CAD build for the part. Positions are in the model's coordinates, mm. Face numbers are marked on the shaded views. Give positions to 0.01 mm unless a question says otherwise; leave off trailing zeros. Loops run counter-clockwise (first coordinate to the right, second up) from the corner with the lowest first, then second, coordinate; pieces in that order, holes last. Notation, with made-up numbers: M -35,86 L 16,86 A12 ccw 16,106 Z; hole C 74.25,-38.75 d7. An arc over 180 degrees is marked long. One line per question, with ' | ' between items.
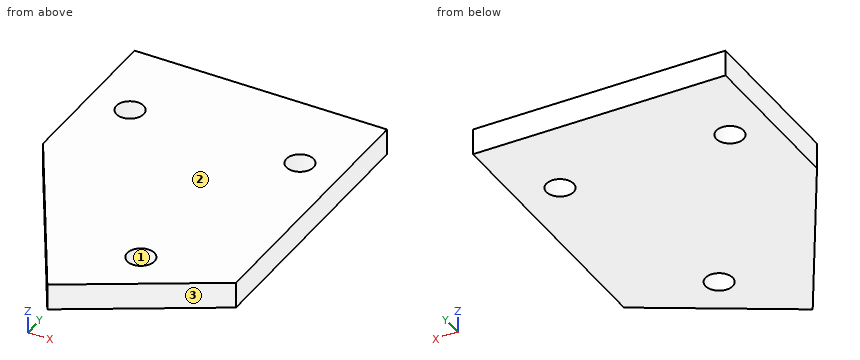
```python
from build123d import *

# Parameters (mm, degrees)
SKETCH1_R           = 1.65
BOSS_EXTRUDE1_DEPTH = 3.175


with BuildPart() as part:
    # Sketch1 → Boss-Extrude1 (new body)
    with BuildSketch(Plane.XY):
        Polygon((0, 0), (13.273502692, -22.990381057), (30.594010768, -12.990381057), (30.594010768, 20), (0, 20), align=None)
        with Locations((19.43375673, -13.660254038)):
            Circle(SKETCH1_R, mode=Mode.SUBTRACT)
        with Locations((5, 10)):
            Circle(SKETCH1_R, mode=Mode.SUBTRACT)
        with Locations((25.594010768, 10)):
            Circle(SKETCH1_R, mode=Mode.SUBTRACT)
    extrude(amount=BOSS_EXTRUDE1_DEPTH)


solid = part.part
```
Item 1: Saw through at A-A on y = 10. Give the cut face in (x, z) (3 decimals).
Conclusion:
outline: M 0,0 L 3.35,0 L 3.35,3.175 L 0,3.175 Z; M 6.65,0 L 23.944,0 L 23.944,3.175 L 6.65,3.175 Z; M 27.244,0 L 30.594,0 L 30.594,3.175 L 27.244,3.175 Z
Item 2: Saw through at D-D on y = -19. Give the cut face in (x, z) (3 decimals).
Conclusion:
outline: M 10.97,0 L 20.185,0 L 20.185,3.175 L 10.97,3.175 Z
Item 3: Saw through at B-B on z = 1.8. Give the cut face in (x, y), and give its area (3 significant figures).
Conclusion:
outline: M 0,0 L 13.27,-22.99 L 30.59,-12.99 L 30.59,20 L 0,20 Z; hole C 5,10 d3.3; hole C 19.43,-13.66 d3.3; hole C 25.59,10 d3.3 | area: 1,050 mm²
Item 4: Saw through at C-C on x = 5. Give the cut face in (y, z) (3 decimals), and give its area (3 significant figures).
Conclusion:
outline: M -8.66,0 L 8.35,0 L 8.35,3.175 L -8.66,3.175 Z; M 11.65,0 L 20,0 L 20,3.175 L 11.65,3.175 Z | area: 80.5 mm²
Item 5: Drill centre lines: line 1 along X through (y, z) = (10.5, 1.75); line 2 along Y through (x, z) = (25, 0.7); line 3 along X through (y, z) = (-13, 0.55). Where is each one in solid material? Low to high. Write a range as [from, to].
Conclusion:
line 1: [0, 3.43], [6.57, 24.02], [27.17, 30.59] | line 2: [-16.22, 8.46], [11.54, 20] | line 3: [7.51, 17.92], [20.95, 30.58]
Item 6: Drop flat-ended pins along their axis: P1, Ø1, axis at x = 21.5, z = 2.5, coming from the -Y side; P2, Ø1, axis at x = 25.5, z = 1, coming from the -Y side; P3, Ø2, axis at x = 19.43, y = -13.66, coming from the -Z side. Give the stop position or say it passes through.
Conclusion:
P1: y = -18.53 | P2: y = -16.22 | P3: through
Item 7: Mould opens along Y. For the marked faces 1, 2 and 3 say: pulls with the +Y half, pulls with the -Y half, needs draft (parallel to the pull), parting line crosses it, or undercut.
Conclusion:
face 1: undercut | face 2: needs draft | face 3: pulls with the -Y half
